Autodesk Inventor part; units mm, degrees
ref_plane "YZ Plane" through (0, 0, 0) normal (1, 0, 0) x (0, 1, 0)
ref_plane "XZ Plane" through (0, 0, 0) normal (0, 1, 0) x (-1, 0, 0)
ref_plane "XY Plane" through (0, 0, 0) normal (0, 0, 1) x (1, 0, 0)
sketch "Sketch1" plane through (0, 0, 0) normal (0, 0, 1) x (1, 0, 0)
  circle A0 centre (0, 0) radius 8
  circle A1 centre (0, 0) radius 15
  dimension "d0" = 16
  dimension "d1" = 30
extrude "Extrusion1" add sketch "Sketch1" along normal blind 3
sketch "Sketch2" plane through (0, 0, 3) normal (0, 0, 1) x (1, 0, 0)
  circle A0 centre (0, 0) radius 8.0485
  circle A1 centre (0, 0) radius 10
  dimension "d4" = 20
extrude "Extrusion2" add sketch "Sketch2" along normal blind 3
properties part number "bushing_1"
The model under review builds one solid part; all positions refer to its coordinate system, in mm. A direction names the side the tool comes from. Give positions to 0.01 mm unless a question says otherwise; leave off trailing zeros. Loops run counter-clockwise (first coordinate to the right, second up) from the corner with the lowest first, then second, coordinate; pieces in that order, holes last. Notation, with made-up numbers: (4, 81) -> (22, 81) arc R30 cw to (22, 109) -> close; hole circle Ø8 at (38, -21). An arc over 180 degrees is marked (long way). Put each result on its own line as item: value. Start each with the question number.
1. For faces 4 (the face through (0.7, 8.2, 6)), 5 (the face through (3, -10, 3)), list the 3-axis set-ups (+Z, -Z, +X, -X, +Y, -Y) from which the entire face can be reached by the end or side of a thin tool; tool diameter is ignored.
2. We need section D-D on y = -9.5. State the section outline as (x, z) points, then the cut area to 3 significant figures.
3. We need section C-C on z = 0.6. State the section outline as (x, y) points.
4. Mouldability with a two-part tool opening along Y and no side actions: class faces 1 (the face through (-2.17, 9.76, 4.48)), 2 (the face through (-1.73, 7.81, 1.48)), 3 (the face through (6, -6, 0)) as released by +Y, released by -Y, zero draft, split by the parting line, or undercut.
5. Clearance check with flat-ended pins moving along their axes: P1, Ø3, axis at x = -9, z = 1.5, coming from the -Y side; P2, Ø3, axis at x = 3, z = 2, coming from the -Y side; P3, Ø1, axis at x = -6.5, z = 2, coming from the +Y side. State where each tip first meets the part, or that it passes through.
6. Wall thickness on probe 1 along Y at (x, z) = (0, 4.7); probe 2 along X at (y, z) = (0.25, 4.5); probe 3 along Z at (x, y) = (1.75, -12): over which ranges is each line inside the solid? List them lowest first.
7. We need section A-A on y = 0. State the section outline as (x, z) points, then the cut area to 3 significant figures.
Determined:
1. face 4: +Z, +X, -X, +Y, -Y
1. face 5: +Z
2. outline: (-11.61, 0) -> (11.61, 0) -> (11.61, 3) -> (3.12, 3) -> (3.12, 6) -> (-3.12, 6) -> (-3.12, 3) -> (-11.61, 3) -> close
2. area: 88.4 mm^2
3. outline: circle Ø30 at (0, 0); hole circle Ø16 at (0, 0)
4. face 1: split by the parting line
4. face 2: undercut
4. face 3: zero draft
5. P1: y = -12.99
5. P2: y = -14.92
5. P3: y = 13.75
6. probe 1: -10 to -8.05, 8.05 to 10
6. probe 2: -10 to -8.04, 8.04 to 10
6. probe 3: 0 to 3
7. outline: (-15, 0) -> (-8, 0) -> (-8, 3) -> (-8.05, 3) -> (-8.05, 6) -> (-10, 6) -> (-10, 3) -> (-15, 3) -> close; (8, 0) -> (15, 0) -> (15, 3) -> (10, 3) -> (10, 6) -> (8.05, 6) -> (8.05, 3) -> (8, 3) -> close
7. area: 53.7 mm^2
